Work out the finished part from the listing and answer in its coordinate system (mm). Face numbers are marked on the shaded views. A direction names the side the tool comes from. Coordinates: 2 decimals unless noted, no trailing zeros. Loops run counter-clockwise (first coordinate to the right, second up) from the corner with the lowest first, then second, coordinate; pieces in that order, holes last.
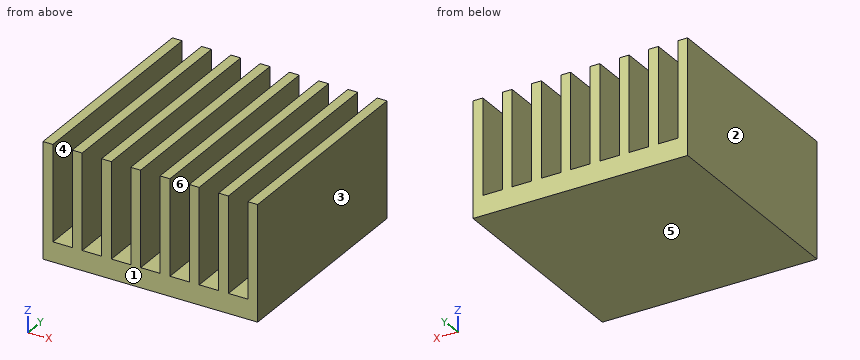
```python
from build123d import *

# Parameters (mm, degrees)
F0_W     = 16.5862
F0_H     = 16.51
F1_DEPTH = 8.89
F2_W     = 1.4986
F2_H     = 7.366
F3_DEPTH = 25.4


with BuildPart() as f1:
    # F0 (on Top) → F1 (new body)
    with BuildSketch(Plane.XY):
        Rectangle(F0_W, F0_H)
    extrude(amount=F1_DEPTH)

    # F2 (on face) → F3 (cut)
    with BuildSketch(Plane.XZ.offset(8.255)):
        with Locations((0, 5.207)):
            Rectangle(F2_W, F2_H)
        with Locations((2.2606, 5.207)):
            Rectangle(F2_W, F2_H)
        with Locations((4.5212, 5.207)):
            Rectangle(F2_W, F2_H)
        with Locations((6.7818, 5.207)):
            Rectangle(F2_W, F2_H)
        with Locations((-2.2606, 5.207)):
            Rectangle(F2_W, F2_H)
        with Locations((-4.5212, 5.207)):
            Rectangle(F2_W, F2_H)
        with Locations((-6.7818, 5.207)):
            Rectangle(F2_W, F2_H)
    extrude(amount=-F3_DEPTH, mode=Mode.SUBTRACT)


solid = f1.part
```
1. A cutting plane is placed at A-A, the plane z = 2.75. Count the separate pieces of the cut face and the enclosed holes in it, then the cut area to 3 significant figures.
2. Determine the mould class of the marked faces 1, 2, 3 and 4 for opening direction X: released by +X, released by -X, zero draft, split by the parting line, or undercut.
3. A straight line is drawn through the part: probe 1 along Z at (x, y) = (-7.5, -7.5). Find the intervals that lie inside material, in ascending order.
4. A cutting plane is placed at C-C, the plane x = 0. Give the vertices of the cut face in (y, z) (3 decimals).
5. For the marked faces 5 and 6, determine the directions among +Z, -Z, +X, -X, +Y, -Y from which every point of the face is accessible in a straight line to the end or side of a thin tool.
6. This flat-tipped pin is pushed along its axis until it touches: P1, Ø1, axis at x = 4.5, y = 3, coming from the +Z side. Where does it stop, or does it pass through?
Answers below:
1. separate pieces: 8
1. enclosed holes: 0
1. area: 101 mm2
2. face 1: zero draft
2. face 2: released by -X
2. face 3: released by +X
2. face 4: undercut
3. probe 1: z = 0 to 1.52
4. outline: (-8.255, 0) - (8.255, 0) - (8.255, 1.524) - (-8.255, 1.524) - close
5. face 5: -Z, +X, -X, +Y, -Y
5. face 6: +Z, +Y, -Y
6. P1: stops at z = 1.52
